Could you check a few things on this model? Use its own coordinates, in mm. Face numbers are marked on the shaded views. A direction names the side the tool comes from. Round coordinates to 2 decimals unless told otherwise and drop trailing zeros. Write each loop counter-clockwise with the first axis right and the second up, starting at its lowest first coordinate (ties: lowest second). Pieces come first, ordered by that corner, then holes.
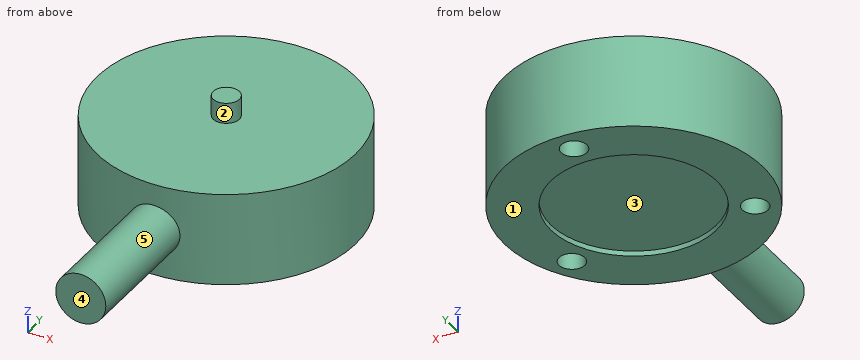
```python
from build123d import *

# Parameters (mm, degrees)
F0_R     = 12.5
F0_R_2   = 1.25
F0_R_3   = 8
F0_R_4   = 1.27
F1_DEPTH = 9
F2_DEPTH = 11
F3_DEPTH = 0.5
F4_DEPTH = 5
F5_R     = 2.425
F6_DEPTH = 25


with BuildPart() as f1:
    # F0 (on Top) → F1 (new body)
    with BuildSketch(Plane.XY):
        Circle(F0_R)
        with Locations((-8.87676, -5.125)):
            Circle(F0_R_2, mode=Mode.SUBTRACT)
        with Locations((8.87676, -5.125)):
            Circle(F0_R_2, mode=Mode.SUBTRACT)
        Circle(F0_R_3, mode=Mode.SUBTRACT)
        with Locations((0, 10.25)):
            Circle(F0_R_2, mode=Mode.SUBTRACT)
        Circle(F0_R_3)
        Circle(F0_R_4, mode=Mode.SUBTRACT)
        with Locations((-8.87676, -5.125)):
            Circle(F0_R_2)
        with Locations((8.87676, -5.125)):
            Circle(F0_R_2)
        Circle(F0_R_4)
        with Locations((0, 10.25)):
            Circle(F0_R_2)
    extrude(amount=F1_DEPTH)

    # F0 (on Top) → F2 (join)
    with BuildSketch(Plane.XY):
        Circle(F0_R_4)
    extrude(amount=F2_DEPTH)

    # F0 (on Top) → F3 (cut)
    with BuildSketch(Plane.XY):
        Circle(F0_R_3)
        Circle(F0_R_4, mode=Mode.SUBTRACT)
        Circle(F0_R_4)
    extrude(amount=F3_DEPTH, mode=Mode.SUBTRACT)

    # F0 (on Top) → F4 (cut)
    with BuildSketch(Plane.XY):
        with Locations((-8.87676, -5.125)):
            Circle(F0_R_2)
        with Locations((8.87676, -5.125)):
            Circle(F0_R_2)
        with Locations((0, 10.25)):
            Circle(F0_R_2)
    extrude(amount=F4_DEPTH, mode=Mode.SUBTRACT)

    # F5 (on Front) → F6 (join)
    with BuildSketch(Plane.XZ):
        with Locations((0, 4.5)):
            Circle(F5_R)
    extrude(amount=F6_DEPTH)


solid = f1.part
```
Q1. On a 3-axis mill with a long thin cutter (end or side, diameter ignored), from which of +Z, -Z, +X, -X, +Y, -Y can I reach the whole of each face in a straight line? I mean the marked faces 4 and 5. Say none if no direction works.
Q2. If I drill on L1, parallel to Y at x = 0, z = 0.4; L2, parallel to Z at x = 7.5, y = 3.5; L3, parallel to X at y = -4.5, z = 2.75, over which ranges is the centre line in solid material (lowest first)?
Q3. Imagine slicing it at A-A, the plane z = 2.5. Write out the boundary of the cut face in (x, y) (3 decimals), then the cut area to 4 significant figures.
Q4. Imagine slicing it at C-C, the plane y = 0. Write out the boundary of the cut face in (x, z).
Q5. I'm going to push flat-ended pins straight in: pin 1 Ø4 at (x, y) = (-9.5, 7.5) entering from +Z; pin 2 Ø1 at (y, z) = (-0.5, 8) entering from +X; pin 3 Ø0.8 at (x, y) = (9, -5.5) entering from -Z; pin 4 Ø5 at (x, z) = (9.5, 8) entering from -Y. Where does each tip first touch, or does it pass through?
Q6. Imagine slicing it at B-B, the plane x = 0. Write out the boundary of the cut face in (y, z) (3 decimals), then the cut area to 3 significant figures.
Q7. Imagine slicing it at D-D, the plane y = 5.5. Write out the boundary of the cut face in (x, z).
Q8. We'd pull the mould along Y, two halves only. Please class the marked faces 1, 2 and 3: pulls with the +Y half, pulls with the -Y half, needs draft (parallel to the pull), parting line crosses it, or undercut.
Results found:
1. face 4: +Z, -Z, +X, -X, -Y
1. face 5: -Y
2. L1: y = -12.5 to -8, 8 to 9, 11.5 to 12.5
2. L2: z = 0 to 9
2. L3: x = -11.66 to -9.96, -7.79 to 7.79, 9.96 to 11.66
3. outline: (-1.371, -25) - (1.371, -25) - (1.371, -12.425) arc R12.5 ccw (long way) to (-1.371, -12.425) - close; hole circle Ø2.5 at (-8.877, -5.125); hole circle Ø2.5 at (0, 10.25); hole circle Ø2.5 at (8.877, -5.125)
3. area: 510.5 mm2
4. outline: (-12.5, 0) - (-8, 0) - (-8, 0.5) - (8, 0.5) - (8, 0) - (12.5, 0) - (12.5, 9) - (1.27, 9) - (1.27, 11) - (-1.27, 11) - (-1.27, 9) - (-12.5, 9) - close
5. pin 1: stops at z = 9
5. pin 2: stops at x = 12.5
5. pin 3: stops at z = 5
5. pin 4: stops at y = -10.36
6. outline: (-25, 2.075) - (-12.5, 2.075) - (-12.5, 0) - (-8, 0) - (-8, 0.5) - (8, 0.5) - (8, 0) - (9, 0) - (9, 5) - (11.5, 5) - (11.5, 0) - (12.5, 0) - (12.5, 9) - (1.27, 9) - (1.27, 11) - (-1.27, 11) - (-1.27, 9) - (-12.5, 9) - (-12.5, 6.925) - (-25, 6.925) - close
6. area: 270 mm2
7. outline: (-11.22, 0) - (-5.81, 0) - (-5.81, 0.5) - (5.81, 0.5) - (5.81, 0) - (11.22, 0) - (11.22, 9) - (-11.22, 9) - close
8. face 1: needs draft
8. face 2: parting line crosses it
8. face 3: undercut
